from build123d import *

# Parameters (mm, degrees)
SKETCH1_R           = 2.4
BOSS_EXTRUDE1_DEPTH = 3


with BuildPart() as part:
    # Sketch1 → Boss-Extrude1 (new body)
    with BuildSketch(Plane(origin=(0, 0, 0), x_dir=(1, 0, 0), z_dir=(0, 1, 0))):
        with BuildLine():
            Line((-18.5, 10), (18.5, 10))
            ThreePointArc((18.5, 10), (19.560660172, 9.560660172), (20, 8.5))
            Line((20, 8.5), (20, -40))
            Line((20, -40), (-20, -40))
            Line((-20, -40), (-20, 8.5))
            ThreePointArc((-20, 8.5), (-19.560660172, 9.560660172), (-18.5, 10))
        make_face()
        with Locations(Location((-10, 0, 0), (0, 0, 270))):
            Circle(SKETCH1_R, mode=Mode.SUBTRACT)
        with Locations(Location((10, 0, 0), (0, 0, 270))):
            Circle(SKETCH1_R, mode=Mode.SUBTRACT)
        with Locations(Location((0, -32.5, 0), (0, 0, 270))):
            Circle(SKETCH1_R, mode=Mode.SUBTRACT)
        with Locations(Location((0, -17.5, 0), (0, 0, 270))):
            Circle(SKETCH1_R, mode=Mode.SUBTRACT)
    extrude(amount=BOSS_EXTRUDE1_DEPTH)


solid = part.part
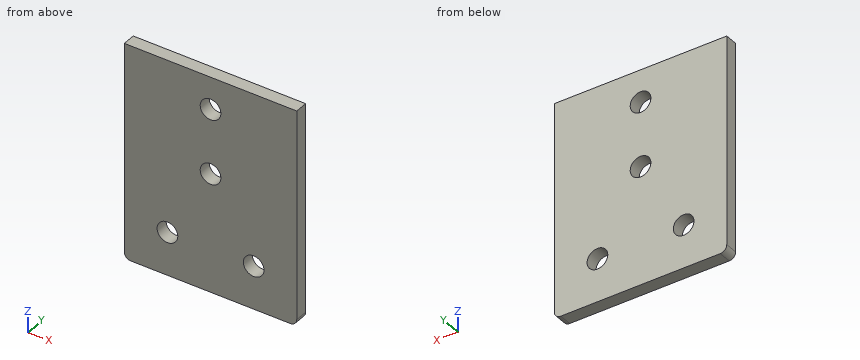
Input: part model. Units: mm. Frame: model coordinates. Give positions to 0.01 mm unless a question says otherwise; leave off trailing zeros. Order: outer loops, then holes, each group sorted by start corner. A loop starts at its lowest first (then second) coordinate and runs counter-clockwise, first axis right, second up. Notation, with made-up numbers: M 49,82.25 L 54,82.25 A16 ccw 54,86.25 Z; hole C 56.25,30 d5. An arc over 180 degrees is marked long. Answer as a JSON object with one key per item and string values.
1. Ray query, line 1 (X direction, y = 0.95, z = 0); line 2 (X direction, y = 2.2, z = 17.5); line 3 (X direction, y = 0.45, z = -1). Return the intervals inside material, ascending. Write a range as [from, to].
Result sheet:
{"line 1": "[-20, -12.4], [-7.6, 7.6], [12.4, 20]", "line 2": "[-20, -2.4], [2.4, 20]", "line 3": "[-20, -12.18], [-7.82, 7.82], [12.18, 20]"}
2. Cut plane A-A, the plane x = -10. Output: boundary loops of the cut face in (y, z), and give its area (3 significant figures).
Result sheet:
{"outline": "M 0,-10 L 3,-10 L 3,-2.4 L 0,-2.4 Z; M 0,2.4 L 3,2.4 L 3,40 L 0,40 Z", "area": "136 mm²"}
3. Cut plane D-D, the plane y = 0.5. Output: boundary loops of the cut face in (x, z).
Result sheet:
{"outline": "M -20,-8.5 A1.5 ccw -18.5,-10 L 18.5,-10 A1.5 ccw 20,-8.5 L 20,40 L -20,40 Z; hole C -10,0 d4.8; hole C 0,17.5 d4.8; hole C 0,32.5 d4.8; hole C 10,0 d4.8"}
4. Cut plane B-B, the plane x = 0. Output: boundary loops of the cut face in (y, z), and give its area (3 significant figures).
Result sheet:
{"outline": "M 0,-10 L 3,-10 L 3,15.1 L 0,15.1 Z; M 0,19.9 L 3,19.9 L 3,30.1 L 0,30.1 Z; M 0,34.9 L 3,34.9 L 3,40 L 0,40 Z", "area": "121 mm²"}
5. Cut plane C-C, the plane z = 0. Output: boundary loops of the cut face in (x, y).
Result sheet:
{"outline": "M -20,0 L -12.4,0 L -12.4,3 L -20,3 Z; M -7.6,0 L 7.6,0 L 7.6,3 L -7.6,3 Z; M 12.4,0 L 20,0 L 20,3 L 12.4,3 Z"}
